Answer from the drawing. Dimensions are ordinates in mm from the lowest x, y and z of the part. A direction names the side the tool comes from. Round coordinates to 2 decimals unless told otherwise and drop trailing zeros. Order: outer loops, then holes, each group sorted by start corner. A loop starts at its lowest first (then second) coordinate and runs counter-clockwise, first axis right, second up.
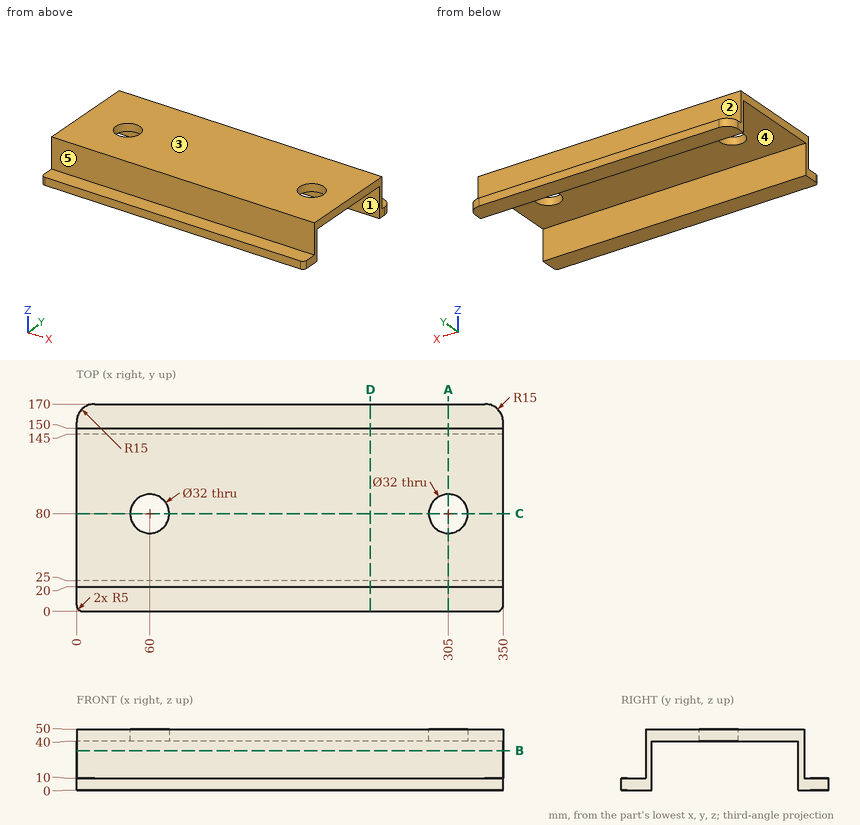
Q1. A cutting plane is placed at C-C, the plane y = 80. Give the vertices of the cut face in (x, z), plus the area to 3 significant figures.
Outcome:
outline: (0, 40) - (44, 40) - (44, 50) - (0, 50) - close; (76, 40) - (289, 40) - (289, 50) - (76, 50) - close; (321, 40) - (350, 40) - (350, 50) - (321, 50) - close
area: 2,860 mm2
Q2. For a pull along Y with two mould halves and no side action, classify the marked faces 3, 4 and 5 as released by +Y, released by -Y, zero draft, split by the parting line, or undercut.
Outcome:
face 3: zero draft
face 4: undercut
face 5: released by -Y
Q3. A cutting plane is placed at B-B, the plane z = 32.5. Give the vertices of the cut face in (x, y).
Outcome:
outline: (0, 20) - (350, 20) - (350, 25) - (0, 25) - close; (0, 145) - (350, 145) - (350, 150) - (0, 150) - close
Q4. A cutting plane is placed at A-A, the plane x = 305. Give the vertices of the cut face in (y, z), plus the area to 3 significant figures.
Outcome:
outline: (0, 0) - (25, 0) - (25, 40) - (64, 40) - (64, 50) - (20, 50) - (20, 10) - (0, 10) - close; (96, 40) - (145, 40) - (145, 0) - (170, 0) - (170, 10) - (150, 10) - (150, 50) - (96, 50) - close
area: 1,780 mm2
Q5. Flat-ended cylindrical pins translate along their axes: pin 1 (1.5 mm diameter, centred on x = 71, y = 113, fed in from -Z); pin 2 (8 mm diameter, centred on x = 186.5, z = 43.5, fed in from +Y); pin 3 (16 mm diameter, centred on x = 190, y = 163, fed in from +Z); pin 4 (5 mm diameter, centred on y = 121, z = 42, fed in from -X). Find the tip coordinate at first contact, or state that the pin passes through.
Outcome:
pin 1: stops at z = 40
pin 2: stops at y = 150
pin 3: stops at z = 10
pin 4: stops at x = 0
Q6. For the marked faces 1 and 2, determine the directions among +Z, -Z, +X, -X, +Y, -Y from which every point of the face is accessible in a straight line to the end or side of a thin tool.
Outcome:
face 1: -Z, +X, -X
face 2: +Z, +X, -X, +Y
Q7. Straight lines are drawn through the part: probe 1 along Y at (x, z) = (255, 36); probe 2 along Y at (x, z) = (60, 47.75); probe 3 along Z at (x, y) = (248, 76.5). For each, find the intervals that lie inside material, in ascending order.
Outcome:
probe 1: y = 20 to 25, 145 to 150
probe 2: y = 20 to 64, 96 to 150
probe 3: z = 40 to 50
Q8. A cutting plane is placed at D-D, the plane x = 241. Give the vertices of the cut face in (y, z), plus the area to 3 significant figures.
Outcome:
outline: (0, 0) - (25, 0) - (25, 40) - (145, 40) - (145, 0) - (170, 0) - (170, 10) - (150, 10) - (150, 50) - (20, 50) - (20, 10) - (0, 10) - close
area: 2,100 mm2
